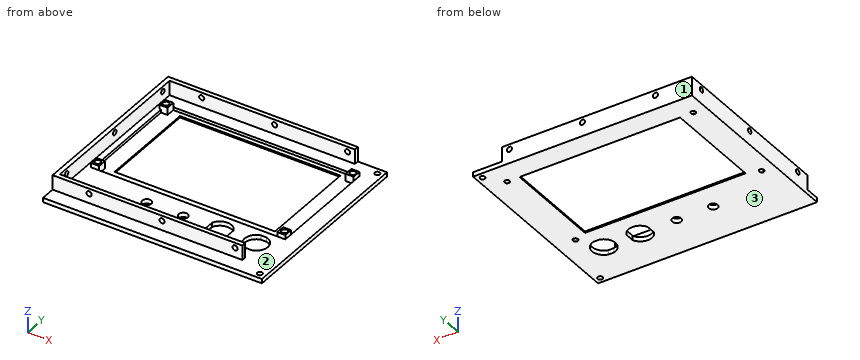
from build123d import *

# Parameters (mm, degrees)
SKETCH_W        = 150
SKETCH_H        = 130
SKETCH_R        = 1.75
SKETCH_W_2      = 110
SKETCH_H_2      = 68
PAD_DEPTH       = 3
SKETCH002_W     = 132
SKETCH002_H     = 77
POCKET001_DEPTH = 2.5
SKETCH007_W     = 5.5
SKETCH007_H     = 6
SKETCH007_R     = 2
PAD002_DEPTH    = 6
PAD003_DEPTH    = 10
SKETCH010_R     = 1.75
POCKET002_DEPTH = 6
SKETCH011_R     = 1.75
POCKET003_DEPTH = 7.5
SKETCH012_R     = 1.75
POCKET004_DEPTH = 7.5
SKETCH015_R     = 8
SKETCH015_R_2   = 3.1
POCKET_DEPTH    = 13.001
SKETCH016_W     = 3.968626
SKETCH016_H     = 0.25
SKETCH016_W_2   = 0.7
SKETCH016_H_2   = 6.545228
PAD004_DEPTH    = 3


with BuildPart() as part:
    # Sketch → Pad (new body)
    with BuildSketch(Plane.XY):
        with Locations((-75, -5)):
            Rectangle(SKETCH_W, SKETCH_H)
        with Locations((-141, 45)):
            Circle(SKETCH_R, mode=Mode.SUBTRACT)
        with Locations((-141, -26)):
            Circle(SKETCH_R, mode=Mode.SUBTRACT)
        with Locations((-13.5, 45)):
            Circle(SKETCH_R, mode=Mode.SUBTRACT)
        with Locations((-13.5, -26)):
            Circle(SKETCH_R, mode=Mode.SUBTRACT)
        with Locations((-4, 56)):
            Circle(SKETCH_R, mode=Mode.SUBTRACT)
        with Locations((-4, -66)):
            Circle(SKETCH_R, mode=Mode.SUBTRACT)
        with Locations((-77, 11)):
            Rectangle(SKETCH_W_2, SKETCH_H_2, mode=Mode.SUBTRACT)
    extrude(amount=PAD_DEPTH)

    # Sketch002 → Pocket001 (cut)
    with BuildSketch(Plane.XY.offset(3.5)):
        with Locations((-77, 9.5)):
            Rectangle(SKETCH002_W, SKETCH002_H)
    extrude(amount=-POCKET001_DEPTH, mode=Mode.SUBTRACT)

    # Sketch007 → Pad002 (join)
    with BuildSketch(Plane.XY):
        with Locations((-141.25, 45)):
            Rectangle(SKETCH007_W, SKETCH007_H)
        with Locations((-141.5, 45)):
            Circle(SKETCH007_R, mode=Mode.SUBTRACT)
        with Locations((-13.75, 45)):
            Rectangle(SKETCH007_W, SKETCH007_H)
        with Locations((-13.5, 45)):
            Circle(SKETCH007_R, mode=Mode.SUBTRACT)
        with Locations((-13.75, -26)):
            Rectangle(SKETCH007_W, SKETCH007_H)
        with Locations((-13.5, -26)):
            Circle(SKETCH007_R, mode=Mode.SUBTRACT)
        with Locations((-141.25, -26)):
            Rectangle(SKETCH007_W, SKETCH007_H)
        with Locations((-141.5, -26)):
            Circle(SKETCH007_R, mode=Mode.SUBTRACT)
    extrude(amount=PAD002_DEPTH)

    # Sketch003 (on DatumPlane) → Pad003 (join)
    with BuildSketch(Plane.XY.offset(3)):
        Polygon((-20, 60), (-150, 60), (-150, -60), (-20, -60), (-20, -57), (-147, -57), (-147, 57), (-20, 57), align=None)
    extrude(amount=PAD003_DEPTH)

    # Sketch010 → Pocket002 (cut)
    with BuildSketch(Plane.XZ.offset(60)):
        with Locations((-125, 9.5)):
            Circle(SKETCH010_R)
        with Locations((-25, 9.5)):
            Circle(SKETCH010_R)
        with Locations((-75, 9.5)):
            Circle(SKETCH010_R)
    extrude(amount=-POCKET002_DEPTH, mode=Mode.SUBTRACT)

    # Sketch011 → Pocket003 (cut, symmetric)
    with BuildSketch(Plane.XZ.offset(-60)):
        with Locations((-75, 9.5)):
            Circle(SKETCH011_R)
        with Locations((-25, 9.5)):
            Circle(SKETCH011_R)
        with Locations((-125, 9.5)):
            Circle(SKETCH011_R)
    extrude(amount=POCKET003_DEPTH, both=True, mode=Mode.SUBTRACT)

    # Sketch012 (on DatumPlane) → Pocket004 (cut, symmetric)
    with BuildSketch(Plane.YZ.offset(-150)):
        with Locations((0, 9.5)):
            Circle(SKETCH012_R)
        with Locations((50, 9.5)):
            Circle(SKETCH012_R)
        with Locations((-50, 9.5)):
            Circle(SKETCH012_R)
    extrude(amount=POCKET004_DEPTH, both=True, mode=Mode.SUBTRACT)

    # Sketch015 → Pocket (cut, through all)
    with BuildSketch(Plane(origin=(0, 0, 0), x_dir=(1, 0, 0), z_dir=(0, 0, -1))):
        with Locations((-48, 41)):
            Circle(SKETCH015_R)
        with Locations((-73, 41)):
            Circle(SKETCH015_R_2)
        with Locations((-98, 41)):
            Circle(SKETCH015_R_2)
        with Locations((-23, 41)):
            Circle(SKETCH015_R)
    extrude(amount=-POCKET_DEPTH, mode=Mode.SUBTRACT)

    # Sketch016 (on Face4 of Pocket) → Pad004 (join)
    with BuildSketch(Plane(origin=(0, 0, 0), x_dir=(1, 0, 0), z_dir=(0, 0, -1))):
        with Locations((-23, 48.875)):
            Rectangle(SKETCH016_W, SKETCH016_H)
        with Locations((-23, 33.125)):
            Rectangle(SKETCH016_W, SKETCH016_H)
        with Locations((-55.65, 41)):
            Rectangle(SKETCH016_W_2, SKETCH016_H_2)
        with Locations((-40.35, 41)):
            Rectangle(SKETCH016_W_2, SKETCH016_H_2)
    extrude(amount=-PAD004_DEPTH)


solid = part.part
Geometry check sheet. Reference: the model listing, model coordinates, mm. Face numbers are marked on the shaded views. Give positions to 0.01 mm unless a question says otherwise; leave off trailing zeros. Order: outer loops, then holes, each group sorted by start corner. A loop starts at its lowest first (then second) coordinate and runs counter-clockwise, first axis right, second up.
1. Sectioned sample at C-C (x = -81). Record the boundary of the cut face in (y, z), then the cut area to 3 significant figures.
Completed:
outline: (-70, 0) - (-23, 0) - (-23, 1) - (-29, 1) - (-29, 3) - (-57, 3) - (-57, 13) - (-60, 13) - (-60, 3) - (-70, 3) - close; (45, 0) - (60, 0) - (60, 13) - (57, 13) - (57, 3) - (48, 3) - (48, 1) - (45, 1) - close
area: 228 mm2
2. Sectioned sample at A-A (y = 13.5). Record the boundary of the cut face in (x, z), then the cut area to 3 significant figures.
Completed:
outline: (-150, 0) - (-132, 0) - (-132, 1) - (-143, 1) - (-143, 3) - (-147, 3) - (-147, 13) - (-150, 13) - close; (-22, 0) - (0, 0) - (0, 3) - (-11, 3) - (-11, 1) - (-22, 1) - close
area: 106 mm2
3. Sectioned sample at D-D (x = -125). Record the boundary of the cut face in (y, z), then the cut area to 3 significant figures.
Completed:
outline: (-70, 0) - (-23, 0) - (-23, 1) - (-29, 1) - (-29, 3) - (-57, 3) - (-57, 7.75) - (-60, 7.75) - (-60, 3) - (-70, 3) - close; (-60, 11.25) - (-57, 11.25) - (-57, 13) - (-60, 13) - close; (45, 0) - (60, 0) - (60, 7.75) - (57, 7.75) - (57, 3) - (48, 3) - (48, 1) - (45, 1) - close; (57, 11.25) - (60, 11.25) - (60, 13) - (57, 13) - close
area: 207 mm2
4. Depth check by flat-ended pin: pin 1 (5.5 mm diameter, centred on y = 0, z = 9.5, fed in from +X); pin 2 (2.5 mm diameter, centred on y = -58.5, z = 7.5, fed in from +X); pin 3 (6 mm diameter, centred on y = -21.5, z = 6.5, fed in from +X). Enter the tip coordinate at first touch or a pass-through.
Completed:
pin 1: stops at x = -147
pin 2: stops at x = -20
pin 3: stops at x = -11
5. Scan lines: line 1 (Y direction, x = -141, z = 0.6); line 2 (X direction, y = -26, z = 2.4); line 3 (Y direction, x = -4, z = 0.7). Record each from-to range of solid material in increasing order.
Completed:
line 1: y = -70 to -27.75, -24.25 to 43.25, 46.75 to 60
line 2: x = -150 to -143, -139.5 to -138.5, -16.5 to -15.5, -11.5 to 0
line 3: y = -70 to -67.75, -64.25 to 54.25, 57.75 to 60
6. Sectioned sample at B-B (x = -98). Record the boundary of the cut face in (y, z), then the cut area to 3 significant figures.
Completed:
outline: (-70, 0) - (-44.1, 0) - (-44.1, 3) - (-57, 3) - (-57, 13) - (-60, 13) - (-60, 3) - (-70, 3) - close; (-37.9, 0) - (-23, 0) - (-23, 1) - (-29, 1) - (-29, 3) - (-37.9, 3) - close; (45, 0) - (60, 0) - (60, 13) - (57, 13) - (57, 3) - (48, 3) - (48, 1) - (45, 1) - close
area: 209 mm2
7. Draft check along Y on the marked faces 1, 2 and 3. Enter one of: pulls with the +Y half, pulls with the -Y half, needs draft (parallel to the pull), parting line crosses it, or undercut.
Completed:
face 1: pulls with the +Y half
face 2: undercut
face 3: needs draft
